from build123d import *

# Parameters (mm, degrees)
SKETCH1_R           = 1
BOSS_EXTRUDE1_DEPTH = 1.5


with BuildPart() as part:
    # Sketch1 → Boss-Extrude1 (new body)
    with BuildSketch(Plane(origin=(0, 0, 0), x_dir=(0, 0, -1), z_dir=(1, 0, 0))):
        with BuildLine():
            Line((6.25, 16.157120391), (6.25, 16.769838997))
            ThreePointArc((6.25, 16.769838997), (5.828394576, 17.99811851), (4.741329439, 18.708548718))
            ThreePointArc((4.741329439, 18.708548718), (3.008303165, 19.064105331), (1.25, 19.259478186))
            Line((1.25, 19.259478186), (1.25, 14.24526237))
            ThreePointArc((1.25, 14.24526237), (0, -14.3), (-1.25, 14.24526237))
            Line((-1.25, 14.24526237), (-1.25, 19.259478186))
            ThreePointArc((-1.25, 19.259478186), (-3.008303352, 19.064105301), (-4.741329807, 18.708548625))
            ThreePointArc((-4.741329807, 18.708548625), (-5.828394693, 17.99811836), (-6.25, 16.769838997))
            Line((-6.25, 16.769838997), (-6.25, 16.157120391))
            ThreePointArc((-6.25, 16.157120391), (-6.555342891, 15.094982319), (-7.378137284, 14.357160556))
            ThreePointArc((-7.378137284, 14.357160556), (-5.6e-08, -17.8), (7.378137384, 14.357160508))
            ThreePointArc((7.378137384, 14.357160508), (6.555342921, 15.094982271), (6.25, 16.157120391))
        make_face()
        with Locations((3.75, 16.365864345)):
            Circle(SKETCH1_R, mode=Mode.SUBTRACT)
        with Locations((-3.75, 16.365864345)):
            Circle(SKETCH1_R, mode=Mode.SUBTRACT)
    extrude(amount=BOSS_EXTRUDE1_DEPTH)


solid = part.part
Input: part model. Units: mm. Frame: model coordinates. A direction names the side the tool comes from. Round coordinates to 2 decimals unless told otherwise and drop trailing zeros. Order: outer loops, then holes, each group sorted by start corner. A loop starts at its lowest first (then second) coordinate and runs counter-clockwise, first axis right, second up.
1. Cut plane B-B, the plane z = 3.75. Output: boundary loops of the cut face in (x, y), then the cut area to 3 significant figures.
The answers:
outline: (0, -17.38) - (1.5, -17.38) - (1.5, -13.8) - (0, -13.8) - close; (0, 13.8) - (1.5, 13.8) - (1.5, 15.37) - (0, 15.37) - close; (0, 17.37) - (1.5, 17.37) - (1.5, 18.93) - (0, 18.93) - close
area: 10.1 mm2
2. Cut plane A-A, the plane y = 0. Output: boundary loops of the cut face in (x, z), then the cut area to 3 significant figures.
The answers:
outline: (0, -16.9) - (1.5, -16.9) - (1.5, -14.3) - (0, -14.3) - close; (0, 14.3) - (1.5, 14.3) - (1.5, 16.9) - (0, 16.9) - close
area: 7.81 mm2
3. Cut plane D-D, the plane y = -8. Output: boundary loops of the cut face in (x, z), then the cut area to 3 significant figures.
The answers:
outline: (0, -15.35) - (1.5, -15.35) - (1.5, -11.85) - (0, -11.85) - close; (0, 11.85) - (1.5, 11.85) - (1.5, 15.35) - (0, 15.35) - close
area: 10.5 mm2
4. Set-up query: faces 4 (the face through (1, 17, 1.25)), 5 (the face through (0, -14.3, -2.4)). Return all of +Z, -Z, +X, -X, +Y, -Y with unobstructed straight access to the full face (end or side cutting, diameter ignored); none if empty.
The answers:
face 4: +X, -X, +Y
face 5: +Z, -Z, -X, +Y, -Y
5. Cut plane C-C, the plane x = 0.9. Output: boundary loops of the cut face in (y, z) (3 decimals).
The answers:
outline: (14.245, -1.25) arc R14.3 cw (long way) to (14.245, 1.25) - (19.259, 1.25) arc R19.3 ccw to (18.709, 4.741) arc R2 ccw to (16.77, 6.25) - (16.157, 6.25) arc R2 cw to (14.357, 7.378) arc R16.925 ccw (long way) to (14.357, -7.378) arc R2 cw to (16.157, -6.25) - (16.77, -6.25) arc R2 ccw to (18.709, -4.741) arc R19.3 ccw to (19.259, -1.25) - close; hole circle Ø2 at (16.366, -3.75); hole circle Ø2 at (16.366, 3.75)
6. Mould query, pull axis Z, two halves, no side actions, for faces 1 (the face through (1.5, -14.3, -2.4)), 2 (the face through (0.74, -14.287, -0.611)), 3 (the face through (0.74, -17.788, 0.637)). Classes: released by +Z, released by -Z, zero draft, split by the parting line, or undercut.
The answers:
face 1: zero draft
face 2: undercut
face 3: split by the parting line
7. Material intervals for line 1 (Y direction, x = 1, z = -3.75); line 2 (Z direction, x = 1, y = 0); line 3 (Z direction, x = 0.95, y = -9.5), sorted ascending.
The answers:
line 1: y = -17.38 to -13.8, 13.8 to 15.37, 17.37 to 18.93
line 2: z = -16.9 to -14.3, 14.3 to 16.9
line 3: z = -14.56 to -10.69, 10.69 to 14.56
8. Pin query (flat end, axial travel): P1, Ø1.6, axis at y = 16.37, z = 3.75, coming from the +X side; P2, Ø0.5, axis at x = 0.5, y = 16.5, coming from the +Z side; P3, Ø0.5, axis at x = 1, y = 16.5, coming from the -Z side. Return the tip coordinate at first contact, or that it passes through.
The answers:
P1: passes through
P2: stops at z = 6.25
P3: stops at z = -6.25
